from build123d import *

# Parameters (mm, degrees)
SKETCH1_R           = 2.5
BOSS_EXTRUDE1_DEPTH = 10
SKETCH3_R           = 5.5
CUT_EXTRUDE1_DEPTH  = 4
BOSS_EXTRUDE2_DEPTH = 20
FILLET1_R           = 10
FILLET2_R           = 5


with BuildPart() as part:
    # Sketch1 → Boss-Extrude1 (new body)
    with BuildSketch(Plane(origin=(0, 0, 0), x_dir=(1, 0, 0), z_dir=(0, 1, 0))):
        with BuildLine():
            Line((-18, -20), (-18, 20))
            ThreePointArc((-18, 20), (-14.832854679, 24.980741817), (-8.978985802, 24.225217038))
            ThreePointArc((-8.978985802, 24.225217038), (0, 20.97437581), (8.978985802, 24.225217038))
            ThreePointArc((8.978985802, 24.225217038), (16.350007855, 23.927777936), (16.794778452, 16.564177238))
            ThreePointArc((16.794778452, 16.564177238), (10.984378813, 0), (16.794778452, -16.564177238))
            ThreePointArc((16.794778452, -16.564177238), (16.350007855, -23.927777936), (8.978985802, -24.225217038))
            ThreePointArc((8.978985802, -24.225217038), (0, -20.97437581), (-8.978985802, -24.225217038))
            ThreePointArc((-8.978985802, -24.225217038), (-14.832854679, -24.980741817), (-18, -20))
        make_face()
        with Locations(Location((-12.5, 20, 0), (0, 0, 270))):
            Circle(SKETCH1_R, mode=Mode.SUBTRACT)
        with Locations(Location((12.5, 20, 0), (0, 0, 90))):
            Circle(SKETCH1_R, mode=Mode.SUBTRACT)
        with Locations(Location((12.5, -20, 0), (0, 0, 270))):
            Circle(SKETCH1_R, mode=Mode.SUBTRACT)
        with Locations(Location((-12.5, -20, 0), (0, 0, 90))):
            Circle(SKETCH1_R, mode=Mode.SUBTRACT)
        with Locations(Location((0, 0, 0), (0, 0, 270))):
            Circle(SKETCH1_R, mode=Mode.SUBTRACT)
    extrude(amount=BOSS_EXTRUDE1_DEPTH)

    # Sketch3 → Cut-Extrude1 (cut)
    with BuildSketch(Plane.XZ):
        with Locations(Location((0, 0, 0), (0, 0, 270))):
            Circle(SKETCH3_R)
    extrude(amount=-CUT_EXTRUDE1_DEPTH, mode=Mode.SUBTRACT)

    # Sketch4 → Boss-Extrude2 (add)
    with BuildSketch(Plane(origin=(0, 10, 0), x_dir=(1, 0, 0), z_dir=(0, 1, 0))):
        Polygon((0, 10.15), (-15, 10.15), (-15, 0), (-15, -10.15), (0, -10.15), (0, -13.15), (-18, -13.15), (-18, 0), (-18, 13.15), (0, 13.15), align=None)
    extrude(amount=BOSS_EXTRUDE2_DEPTH)

    # Fillet1
    fillet1_edges = [part.edges().sort_by_distance(p)[0] for p in [
        (0, 10, -11.65),
        (0, 10, 11.65),
    ]]
    fillet(fillet1_edges, radius=FILLET1_R)

    # Fillet2
    fillet2_edges = [part.edges().sort_by_distance(p)[0] for p in [
        (-18, 20, -13.15),
        (-18, 20, 13.15),
    ]]
    fillet(fillet2_edges, radius=FILLET2_R)


solid = part.part
The listing builds one solid part. Answer for the finished solid, in the listing's coordinates (mm). A direction names the side the tool comes from. Give positions to 0.01 mm unless a question says otherwise; leave off trailing zeros. Order: outer loops, then holes, each group sorted by start corner. A loop starts at its lowest first (then second) coordinate and runs counter-clockwise, first axis right, second up. Notation, with made-up numbers: (69.5, 73) - (87.5, 73) arc R11 cw to (87.5, 86) - close; hole circle Ø3 at (1.25, -8). An arc over 180 degrees is marked (long way). Use one line per item in the form item = value.
1) Find section C-C on x = 1. Determine the outline of the cut face in (y, z).
Verdict:
outline = (0, -21.01) - (10, -21.01) - (10, -13.15) - (15.64, -13.15) - (15.64, -10.15) - (10, -10.15) - (10, -2.29) - (4, -2.29) - (4, -5.41) - (0, -5.41) - close; (0, 5.41) - (4, 5.41) - (4, 2.29) - (10, 2.29) - (10, 10.15) - (15.64, 10.15) - (15.64, 13.15) - (10, 13.15) - (10, 21.01) - (0, 21.01) - close
2) Each of these flat-tipped pins is pushed along its axis until it touches: pin 1 (1.5 mm diameter, centred on y = 24.5, z = -11.5, fed in from +X); pin 2 (3 mm diameter, centred on x = 12.5, z = -20, fed in from +Y); pin 3 (1.5 mm diameter, centred on x = -10.5, y = 12.5, fed in from +Z); pin 4 (1.5 mm diameter, centred on x = -3, y = 8, fed in from -Z) (3 decimals). Where does it stop, or does it pass through?
Verdict:
pin_1 = 0
pin_2 = through
pin_3 = 13.15
pin_4 = -21.485
3) The mould has two halves that part along Z. Classify faces 1 (the cylindrical face through (-16.5, 20.14, 11.72)), 2 (the cylindrical face through (-0.136, 4.93, -20.975)), 3 (the cylindrical face through (11, 5, 18)): released by +Z, released by -Z, zero draft, split by the parting line, or undercut.
Verdict:
face_1 = released by +Z
face_2 = released by -Z
face_3 = undercut
4) Find section D-D on y = 27. Determine the outline of the cut face in (x, z), and give its area (3 significant figures).
Verdict:
outline = (-18, -8.15) arc R5 ccw to (-13, -13.15) - (0, -13.15) - (0, -10.15) - (-15, -10.15) - (-15, 10.15) - (0, 10.15) - (0, 13.15) - (-13, 13.15) arc R5 ccw to (-18, 8.15) - close
area = 158 mm^2
5) Find section A-A on z = 0. Determine the outline of the cut face in (x, y), and give its area (3 significant figures).
Verdict:
outline = (-18, 0) - (-5.5, 0) - (-5.5, 4) - (-2.5, 4) - (-2.5, 10) - (-15, 10) - (-15, 30) - (-18, 30) - close; (2.5, 4) - (5.5, 4) - (5.5, 0) - (10.98, 0) - (10.98, 10) - (2.5, 10) - close
area = 276 mm^2
6) For faces 4 (the flat face through (-8, 20, -10.15)), 5 (the flat face through (0, 4, 3)), 6 (the flat face through (0, 25, 12)), determine the directions among +Z, -Z, +X, -X, +Y, -Y from which every point of the face is accessible in a straight line to the end or side of a thin tool.
Verdict:
face_4 = +X, +Y
face_5 = -Y
face_6 = +Z, -Z, +X, +Y
7) Find section B-B on y = 6. Determine the outline of the cut face in (x, z), and give its area (3 significant figures).
Verdict:
outline = (-18, -20) arc R5.5 ccw to (-8.98, -24.23) arc R14.03 cw to (8.98, -24.23) arc R5.5 ccw to (16.79, -16.56) arc R26.52 cw to (16.79, 16.56) arc R5.5 ccw to (8.98, 24.23) arc R14.03 cw to (-8.98, 24.23) arc R5.5 ccw to (-18, 20) - close; hole circle Ø5 at (-12.5, -20); hole circle Ø5 at (-12.5, 20); hole circle Ø5 at (0, 0); hole circle Ø5 at (12.5, -20); hole circle Ø5 at (12.5, 20)
area = 1,410 mm^2
8) Consider probe 1 along X at (y, z) = (4.25, 20); probe 2 along Z at (x, y) = (0, 8.75); probe 3 along Z at (x, y) = (-1.5, 25.25). Determine where each line is inside the solid, lowest interval first. Write a range as [from, to].
Verdict:
probe_1 = [-18, -15], [-10, 10], [15, 18]
probe_2 = [-20.97, -2.5], [2.5, 20.97]
probe_3 = [-13.15, -10.15], [10.15, 13.15]
